Can you work these out from the drawing? Everything is in mm from the part's minimum corner. Coordinates: 2 decimals unless noted, no trailing zeros. Order: outer loops, then holes, each group sorted by start corner. A loop starts at its lowest first (then second) coordinate and runs counter-clockwise, first axis right, second up. Notation, with made-up numbers: (27.5, 38.25) -> (37.5, 38.25) arc R21 cw to (37.5, 43.25) -> close; hole circle Ø11 at (35, 26.5). An arc over 180 degrees is marked (long way). Put each result on its own line as item: value. Start each with the question number.
Q1. We'd pull the mould along Z, two halves only. Please class the marked faces 1 and 2: +Z half, -Z half, draft (parallel to the pull), parting line (faces both ways), or undercut.
Q2. If we section it at A-A (x = 12): Please give me the cut outline in (y, z), and give its area (3 significant figures).
Q3. If we section it at B-B (z = 16.5): Please give me the cut outline in (x, y), and give its area (3 significant figures).
Q4. Will this pin go through, and if not, where does the flat tip stop? pin 1 (7.5 mm diameter, centred on x = 10, z = 19, fed in from -Y).
Q5. Please list where these lines run through material, in increasing order: line 1 along X through (y, z) = (0.3, 9); line 2 along Y through (x, z) = (22, 10).
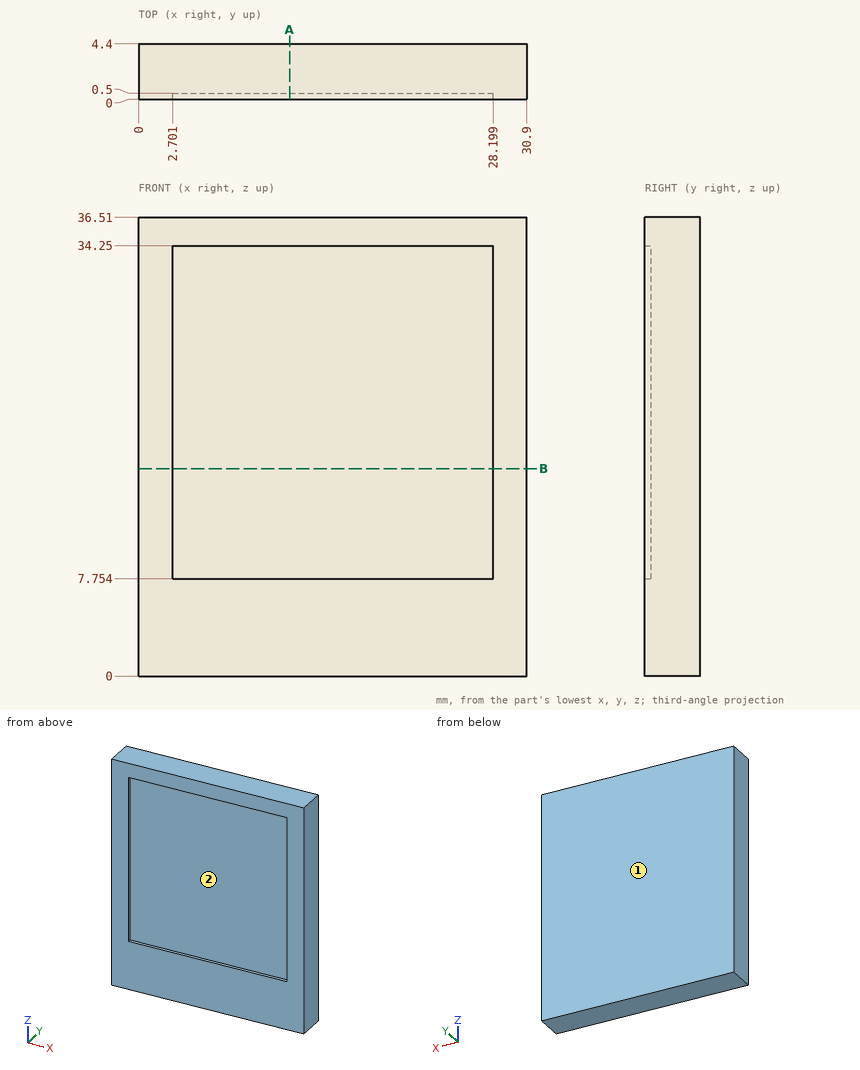
The answers:
1. face 1: draft
1. face 2: undercut
2. outline: (0, 0) -> (4.4, 0) -> (4.4, 36.51) -> (0, 36.51) -> (0, 34.25) -> (0.5, 34.25) -> (0.5, 7.75) -> (0, 7.75) -> close
2. area: 147 mm^2
3. outline: (0, 0) -> (2.7, 0) -> (2.7, 0.5) -> (28.2, 0.5) -> (28.2, 0) -> (30.9, 0) -> (30.9, 4.4) -> (0, 4.4) -> close
3. area: 123 mm^2
4. pin 1: y = 0.5
5. line 1: 0 to 2.7, 28.2 to 30.9
5. line 2: 0.5 to 4.4
